Source: CAD feature listing. Evaluate the final solid. Frame: model axes, mm. Face numbers are marked on the shaded views. A direction names the side the tool comes from. Coordinates: 2 decimals unless noted, no trailing zeros. Write each loop counter-clockwise with the first axis right and the second up, starting at its lowest first coordinate (ties: lowest second). Pieces come first, ordered by that corner, then holes. Notation, with made-up numbers: (-7, 28) - (2, 28) arc R36 cw to (2, 62) - close; hole circle Ø1 at (43.25, 74). An arc over 180 degrees is marked (long way). One line per question, with ' | ' between items.
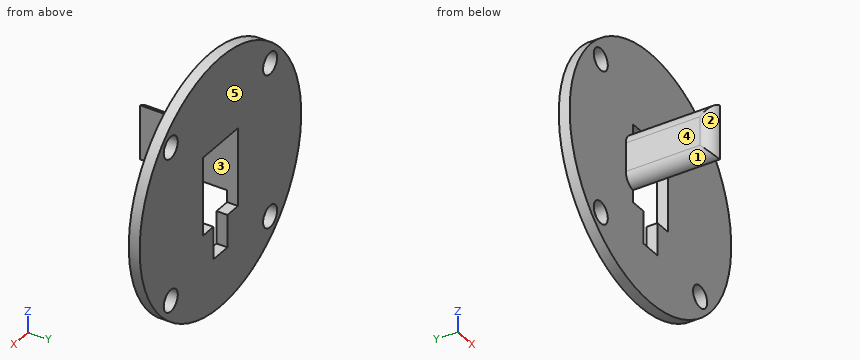
from build123d import *

# Parameters (mm, degrees)
SKETCH2_R           = 57.5
BOSS_EXTRUDE1_DEPTH = 5
SKETCH3_R           = 5
CUT_EXTRUDE1_DEPTH  = 82.470853684
SKETCH4_W           = 25
SKETCH4_H           = 36
CUT_EXTRUDE2_DEPTH  = 82.470853684
SKETCH5_W           = 5
SKETCH5_H           = 25
BOSS_EXTRUDE2_DEPTH = 40
FILLET1_R           = 6
SKETCH7_W           = 10
SKETCH7_H           = 15
CUT_EXTRUDE3_DEPTH  = 93.938151477


with BuildPart() as part:
    # Sketch2 → Boss-Extrude1 (new body)
    with BuildSketch(Plane(origin=(0, 0, 0), x_dir=(1, 0, 0), z_dir=(0, 1, 0))):
        with Locations(Location((0, 0, 0), (0, 0, 270))):
            Circle(SKETCH2_R)
    extrude(amount=BOSS_EXTRUDE1_DEPTH)

    # Sketch3 → Cut-Extrude1 (cut, through all)
    with BuildSketch(Plane(origin=(0, 5, 0), x_dir=(1, 0, 0), z_dir=(0, 1, 0))):
        with Locations(Location((-35.355339059, 35.355339059, 0), (0, 0, 270))):
            Circle(SKETCH3_R)
        with Locations(Location((35.355339059, 35.355339059, 0), (0, 0, 270))):
            Circle(SKETCH3_R)
        with Locations(Location((35.355339059, -35.355339059, 0), (0, 0, 270))):
            Circle(SKETCH3_R)
        with Locations(Location((-35.355339059, -35.355339059, 0), (0, 0, 270))):
            Circle(SKETCH3_R)
    extrude(amount=-CUT_EXTRUDE1_DEPTH, mode=Mode.SUBTRACT)

    # Sketch4 → Cut-Extrude2 (cut, through all)
    with BuildSketch(Plane(origin=(0, 5, 0), x_dir=(1, 0, 0), z_dir=(0, 1, 0))):
        Rectangle(SKETCH4_W, SKETCH4_H)
    extrude(amount=-CUT_EXTRUDE2_DEPTH, mode=Mode.SUBTRACT)

    # Sketch5 → Boss-Extrude2 (add)
    with BuildSketch(Plane.XZ):
        with Locations((-15, 0)):
            Rectangle(SKETCH5_W, SKETCH5_H)
    extrude(amount=BOSS_EXTRUDE2_DEPTH)

    # Fillet1
    # the kernel refuses this fillet: 6 mm, written as the material it takes off along each edge
    with BuildSketch(Plane(origin=(-17.5, -40, 27.290199458), x_dir=(0, 1, 0), z_dir=(0, 0, -1))) as fillet1_piece_1:
        with BuildLine():
            CenterArc((5.916079783, 6), FILLET1_R, 189.594068227, 80.405931773)
            Line((0, 5), (0, 0))
            Line((0, 0), (5.916079783, 0))
        make_face()
    extrude(amount=54.580398916, mode=Mode.SUBTRACT)
    with BuildSketch(Plane(origin=(-17.5, 0, -12.5), x_dir=(1, 0, 0), z_dir=(0, -1, 0))) as fillet1_piece_2:
        with BuildLine():
            CenterArc((6, 5.916079783), FILLET1_R, 180, 80.405931773)
            Line((0, 5.916079783), (0, 0))
            Line((0, 0), (5, 0))
        make_face()
    extrude(amount=54.790199458, mode=Mode.SUBTRACT)
    with BuildSketch(Plane(origin=(-17.5, 0, 12.5), x_dir=(0, 0, -1), z_dir=(0, -1, 0))) as fillet1_piece_3:
        with BuildLine():
            CenterArc((5.916079783, 6), FILLET1_R, 189.594068227, 80.405931773)
            Line((0, 5), (0, 0))
            Line((0, 0), (5.916079783, 0))
        make_face()
    extrude(amount=54.790199458, mode=Mode.SUBTRACT)

    # Sketch7 → Cut-Extrude3 (cut, through all)
    with BuildSketch(Plane(origin=(0, 5, 0), x_dir=(1, 0, 0), z_dir=(0, 1, 0))):
        with Locations((0, 25.5)):
            Rectangle(SKETCH7_W, SKETCH7_H)
    extrude(amount=-CUT_EXTRUDE3_DEPTH, mode=Mode.SUBTRACT)


solid = part.part
Item 1: Ray query, line 1 along X through (y, z) = (-2, -5); line 2 along Y through (x, z) = (17.5, 39.5); line 3 along X through (y, z) = (1, 15). Return the intervals inside material, ascending. Write a range as [from, to].
Check sheet entries:
line 1: [-17.5, -12.5] | line 2: [0, 5] | line 3: [-55.51, -12.5], [12.5, 55.51]
Item 2: Access query for the marked faces 4 and 5. Directions: +Z, -Z, +X, -X, +Y, -Y. A direction counts if a zero-diameter tool reaches every point of the face in a straight line with its end or side. Return the directions, or none.
Check sheet entries:
face 4: +Z, -Z, -X, -Y | face 5: +Z, -Z, +X, -X, +Y
Item 3: Mould query, pull axis Z, two halves, no side actions, for the marked faces 1, 2 and 3. Classes: pulls with the +Z half, pulls with the -Z half, needs draft (parallel to the pull), parting line crosses it, or undercut.
Check sheet entries:
face 1: pulls with the -Z half | face 2: needs draft | face 3: undercut
Item 4: Cut plane C-C on x = 33.5. Return loops of the section in (y, z), and give its area (3 significant figures).
Check sheet entries:
outline: (0, -46.73) - (5, -46.73) - (5, -40) - (0, -40) - close; (0, -30.71) - (5, -30.71) - (5, 30.71) - (0, 30.71) - close; (0, 40) - (5, 40) - (5, 46.73) - (0, 46.73) - close | area: 374 mm²
Item 5: Pin query (flat end, axial travel): pin 1 Ø5.5 at (y, z) = (3.5, -27) entering from +X; pin 2 Ø1.5 at (y, z) = (2, -25.5) entering from -X; pin 3 Ø1.5 at (x, y) = (2.5, 3.5) entering from -Z. Return the tip coordinate at first contact, or that it passes through.
Check sheet entries:
pin 1: x = 52.14 | pin 2: x = -51.9 | pin 3: z = -57.47
Item 6: Cut plane A-A on z = 0. Return loops of the section in (x, y).
Check sheet entries:
outline: (-57.5, 0) - (-17.5, 0) - (-17.5, -34.08) arc R6 ccw to (-12.5, -40) - (-12.5, 5) - (-57.5, 5) - close; (12.5, 0) - (57.5, 0) - (57.5, 5) - (12.5, 5) - close
Item 7: Cut plane D-D on y = -17. Return loops of the section in (x, z).
Check sheet entries:
outline: (-17.5, -6.58) arc R6 ccw to (-12.5, -12.5) - (-12.5, 12.5) arc R6 ccw to (-17.5, 6.58) - close
Item 8: Cut plane B-B on x = 0. Return loops of the section in (y, z).
Check sheet entries:
outline: (0, -57.5) - (5, -57.5) - (5, -33) - (0, -33) - close; (0, 18) - (5, 18) - (5, 57.5) - (0, 57.5) - close
